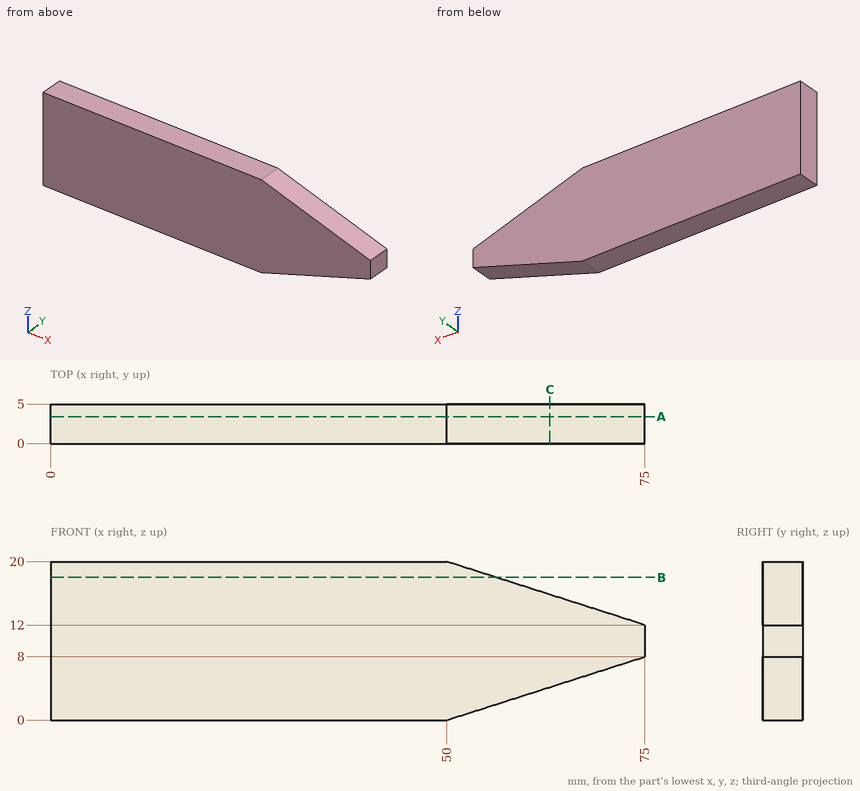
Design review of the part shown in the three views and the two pictorial views. Dimensions are in mm from the part's minimum x, y and z. Round coordinates to 2 decimals unless told otherwise and drop trailing zeros. Order: outer loops, then holes, each group sorted by start corner. A loop starts at its lowest first (then second) coordinate and runs counter-clockwise, first axis right, second up.
(1) For P1, Ø8, axis at x = 22.5, z = 10, coming from the -Y side, flat-tipped, find the tip position at first contact; note if it passes through.
Working result:
P1: stops at y = 0
(2) Wall thickness on L1, parallel to Z at x = 54, y = 3.6; L2, parallel to Z at x = 69.5, y = 3.6: over which ranges is each line inside the solid? List them lowest first.
Working result:
L1: z = 1.28 to 18.72
L2: z = 6.24 to 13.76
(3) Take a section at B-B, the plane z = 18. State the section outline as (x, y) points.
Working result:
outline: (0, 0) - (56.25, 0) - (56.25, 5) - (0, 5) - close
(4) Take a section at A-A, the plane y = 3.4. State the section outline as (x, z) points, plus the area to 3 significant figures.
Working result:
outline: (0, 0) - (50, 0) - (75, 8) - (75, 12) - (50, 20) - (0, 20) - close
area: 1,300 mm2
(5) Take a section at C-C, the plane x = 63. State the section outline as (y, z) points.
Working result:
outline: (0, 4.16) - (5, 4.16) - (5, 15.84) - (0, 15.84) - close
